from build123d import *

# Parameters (mm, degrees)
SKETCH1_R           = 18
SKETCH1_R_2         = 2.6
SKETCH1_R_3         = 1.45
BOSS_EXTRUDE1_DEPTH = 6
SKETCH2_R           = 2.5
CUT_EXTRUDE1_DEPTH  = 2.51
SKETCH3_R           = 7.6
CUT_EXTRUDE2_DEPTH  = 1.2
CUT_EXTRUDE3_DEPTH  = 3.6
SKETCH5_R           = 4.5
SKETCH5_R_2         = 2.6
BOSS_EXTRUDE2_DEPTH = 0.5


with BuildPart() as part:
    # Sketch1 → Boss-Extrude1 (new body)
    with BuildSketch(Plane.XY.offset(322)):
        with Locations((300, 300)):
            Circle(SKETCH1_R)
        with Locations((300, 300)):
            Circle(SKETCH1_R_2, mode=Mode.SUBTRACT)
        with Locations((300, 313.5)):
            Circle(SKETCH1_R_3, mode=Mode.SUBTRACT)
        with Locations((288.308657049, 293.25)):
            Circle(SKETCH1_R_3, mode=Mode.SUBTRACT)
        with Locations((311.691342951, 293.25)):
            Circle(SKETCH1_R_3, mode=Mode.SUBTRACT)
    extrude(amount=BOSS_EXTRUDE1_DEPTH)

    # Sketch2 → Cut-Extrude1 (cut)
    with BuildSketch(Plane.XY.offset(325.5)):
        with Locations((300, 313.5)):
            Circle(SKETCH2_R)
        with Locations((288.308657049, 293.25)):
            Circle(SKETCH2_R)
        with Locations((311.691342951, 293.25)):
            Circle(SKETCH2_R)
    extrude(amount=CUT_EXTRUDE1_DEPTH, mode=Mode.SUBTRACT)

    # Sketch3 → Cut-Extrude2 (cut)
    with BuildSketch(Plane.XY.offset(322)):
        with Locations((300, 300)):
            Circle(SKETCH3_R)
    extrude(amount=CUT_EXTRUDE2_DEPTH, mode=Mode.SUBTRACT)

    # Sketch4 → Cut-Extrude3 (cut)
    with BuildSketch(Plane.XY.offset(323.2)):
        Polygon((304.734272207, 300), (302.367136104, 304.1), (297.632863896, 304.1), (295.265727793, 300), (297.632863896, 295.9), (302.367136104, 295.9), align=None)
    extrude(amount=CUT_EXTRUDE3_DEPTH, mode=Mode.SUBTRACT)

    # Sketch5 → Boss-Extrude2 (add)
    with BuildSketch(Plane.XY.offset(328)):
        with Locations((300, 300)):
            Circle(SKETCH5_R)
        with Locations((300, 300)):
            Circle(SKETCH5_R_2, mode=Mode.SUBTRACT)
    extrude(amount=BOSS_EXTRUDE2_DEPTH)


solid = part.part
For this review, take the finished solid that the model builds, in its own axes (mm). A direction names the side the tool comes from. Coordinates: 2 decimals unless noted, no trailing zeros. Loops run counter-clockwise (first coordinate to the right, second up) from the corner with the lowest first, then second, coordinate; pieces in that order, holes last. Notation, with made-up numbers: (-3.75, 14) - (22.25, 14) arc R21 ccw to (22.25, 49) - close; hole circle Ø5 at (88, 55). An arc over 180 degrees is marked (long way). Use a Markdown table: item, result. Add a question column.
Item 1: Insertion check: pin 1 Ø1 at (y, z) = (308.5, 325) entering from -X; pin 2 Ø7.5 at (x, y) = (303, 302) entering from -Z; pin 3 Ø3 at (x, z) = (290.5, 326) entering from +Y. Each pin has a flat end and moves straight along its axis. Give the tip position at first contact, or say it passes through.
Item 2: For line 1 (X direction, y = 300, z = 328.1); line 2 (Y direction, x = 300, z = 324.15); line 3 (X direction, y = 293.25, z = 324.2), list the stretches that pass through material, from the lowest coordinate up.
Item 3: Mouldability with a two-part tool opening along Y and no side actions: class faces 1 (the face through (302, 298, 328.5)), 2 (the face through (288.3, 291.6, 325.5)), 3 (the face through (297.657, 317.847, 324.958)), 4 (the face through (298.93, 314.48, 323.73)) as pulls with the +Y half, pulls with the -Y half, needs draft (parallel to the pull), parting line crosses it, or undercut.
Item 4: We need section D-D (x = 288). Give the boundary of the cut face in (y, z).
Item 5: Tool access review of faces 5 (the face through (296.466, 302.079, 324.975)), 6 (the face through (311.503, 294.688, 323.726)), 7 (the face through (302.31, 312.54, 326.73)): name each direction out of +Z, -Z, +X, -X, +Y, -Y from which nothing blocks a thin tool from reaching the whole face with its end or side.
Item 6: We need section C-C (y = 313.5). Give the boundary of the cut face in (x, z), and give its area (3 significant figures).
Item 7: We need section B-B (z = 326). Give the boundary of the cut face in (x, y), and give its area (3 significant figures).
Item 8: We need section A-A (x = 300). Give the boundary of the cut face in (y, z), and give its area (3 significant figures).
Results list:
| question | item | result |
|---|---|---|
| 1 | pin 1 | stops at x = 283.88 |
| 1 | pin 2 | stops at z = 323.2 |
| 1 | pin 3 | stops at y = 316.12 |
| 2 | line 1 | x = 295.5 to 297.4, 302.6 to 304.5 |
| 2 | line 2 | y = 282 to 295.9, 304.1 to 312.05, 314.95 to 318 |
| 2 | line 3 | x = 283.31 to 286.86, 289.76 to 310.24, 313.14 to 316.69 |
| 3 | face 1 | needs draft |
| 3 | face 2 | undercut |
| 3 | face 3 | parting line crosses it |
| 3 | face 4 | undercut |
| 4 | outline | (286.58, 322) - (291.83, 322) - (291.83, 325.5) - (290.77, 325.5) - (290.77, 328) - (286.58, 328) - close; (294.67, 322) - (313.42, 322) - (313.42, 328) - (295.73, 328) - (295.73, 325.5) - (294.67, 325.5) - close |
| 5 | face 5 | -Z |
| 5 | face 6 | +Z, -Z |
| 5 | face 7 | +Z |
| 6 | outline | (288.09, 322) - (298.55, 322) - (298.55, 325.5) - (297.5, 325.5) - (297.5, 328) - (288.09, 328) - close; (301.45, 322) - (311.91, 322) - (311.91, 328) - (302.5, 328) - (302.5, 325.5) - (301.45, 325.5) - close |
| 6 | area | 120 mm^2 |
| 7 | outline | circle Ø36 at (300, 300); hole circle Ø5 at (288.31, 293.25); hole (295.27, 300) - (297.63, 295.9) - (302.37, 295.9) - (304.73, 300) - (302.37, 304.1) - (297.63, 304.1) - close; hole circle Ø5 at (300, 313.5); hole circle Ø5 at (311.69, 293.25) |
| 7 | area | 901 mm^2 |
| 8 | outline | (282, 322) - (292.4, 322) - (292.4, 323.2) - (295.9, 323.2) - (295.9, 326.8) - (297.4, 326.8) - (297.4, 328.5) - (295.5, 328.5) - (295.5, 328) - (282, 328) - close; (302.6, 326.8) - (304.1, 326.8) - (304.1, 323.2) - (307.6, 323.2) - (307.6, 322) - (312.05, 322) - (312.05, 325.5) - (311, 325.5) - (311, 328) - (304.5, 328) - (304.5, 328.5) - (302.6, 328.5) - close; (314.95, 322) - (318, 322) - (318, 328) - (316, 328) - (316, 325.5) - (314.95, 325.5) - close |
| 8 | area | 141 mm^2 |
